Could you check a few things on this model? Use its own coordinates, in mm. Face numbers are marked on the shaded views. A direction names the side the tool comes from. Coordinates: 2 decimals unless noted, no trailing zeros. Loops run counter-clockwise (first coordinate to the right, second up) from the corner with the lowest first, then second, coordinate; pieces in that order, holes last.
1) Imagine slicing it at C-C on y = -9.75. Please give me the cut outline in (x, z), plus the area to 4 significant figures.
2) Imagine slicing it at A-A on y = 0. Please give me the cut outline in (x, z).
3) If I drill on line 1 along Y through (x, z) = (0, 14.5); line 2 along Y through (x, z) = (2.5, 14.5); line 3 along Z through (x, y) = (6.75, -6.5), over which ranges is the centre line in solid material (lowest first)?
4) Imagine slicing it at B-B on z = 4.25. Please give me the cut outline in (x, y).
5) For the marked faces 1 and 2, which set-ups out of +Z, -Z, +X, -X, +Y, -Y let a thin tool reach every point of the face, with its end or its side?
6) Will these pins go through, and if not, where does the flat tip stop? P1, Ø1, axis at x = 4, z = 17, coming from the -Y side; P2, Ø3, axis at x = 6.5, z = 6.5, coming from the +Y side; P3, Ø1, axis at x = -4.5, z = 3, coming from the -Y side; P4, Ø6, axis at x = -0.5, y = -0.5, coming from the +Z side.
7) Imagine slicing it at D-D on x = 7.5. Please give me the cut outline in (y, z).
8) Thinking about a two-plate mould opening in X: for the marked faces 3, 4 and 5, which applies, released by +X, released by -X, zero draft, split by the parting line, or undercut?
```python
from build123d import *

# Parameters (mm, degrees)
BOSS_EXTRUDE1_DEPTH = 7.62
SKETCH2_R           = 6.35
BOSS_EXTRUDE2_DEPTH = 12.7
SKETCH3_R           = 3.81
CUT_EXTRUDE1_DEPTH  = 21.32
CHAMFER1_SIZE       = 1.27


with BuildPart() as part:
    # Sketch1 → Boss-Extrude1 (new body)
    with BuildSketch(Plane.XY):
        Polygon((10.31875, 5.95753309), (0, 11.91506618), (-10.31875, 5.95753309), (-10.31875, -5.95753309), (0, -11.91506618), (10.31875, -5.95753309), align=None)
    extrude(amount=BOSS_EXTRUDE1_DEPTH)

    # Sketch2 → Boss-Extrude2 (add)
    with BuildSketch(Plane.XY.offset(7.62)):
        Circle(SKETCH2_R)
    extrude(amount=BOSS_EXTRUDE2_DEPTH)

    # Sketch3 → Cut-Extrude1 (cut, through all)
    with BuildSketch(Plane.XY.offset(20.32)):
        Circle(SKETCH3_R)
    extrude(amount=-CUT_EXTRUDE1_DEPTH, mode=Mode.SUBTRACT)

    # Chamfer1
    chamfer1_edges = [part.edges().sort_by_distance(p)[0] for p in [
        (-3.81, 0, 0),
        (-3.81, 0, 20.32),
    ]]
    chamfer(chamfer1_edges, length=CHAMFER1_SIZE)


solid = part.part
```
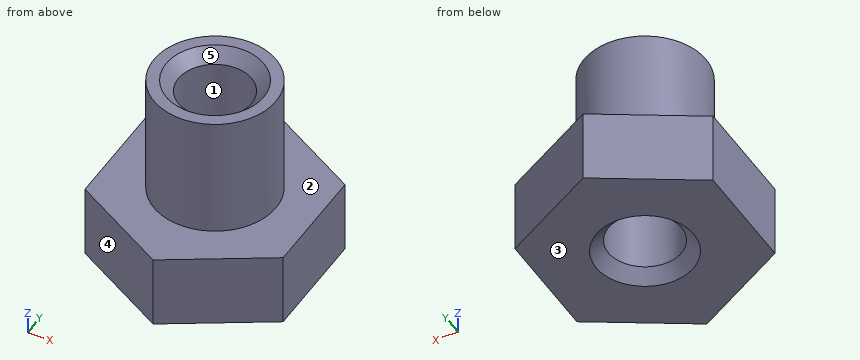
Filled in:
1. outline: (-3.75, 0) - (3.75, 0) - (3.75, 7.62) - (-3.75, 7.62) - close
1. area: 57.15 mm2
2. outline: (-10.32, 0) - (-5.08, 0) - (-3.81, 1.27) - (-3.81, 19.05) - (-5.08, 20.32) - (-6.35, 20.32) - (-6.35, 7.62) - (-10.32, 7.62) - close; (3.81, 1.27) - (5.08, 0) - (10.32, 0) - (10.32, 7.62) - (6.35, 7.62) - (6.35, 20.32) - (5.08, 20.32) - (3.81, 19.05) - close
3. line 1: y = -6.35 to -3.81, 3.81 to 6.35
3. line 2: y = -5.84 to -2.88, 2.88 to 5.84
3. line 3: z = 0 to 7.62
4. outline: (-10.32, -5.96) - (0, -11.92) - (10.32, -5.96) - (10.32, 5.96) - (0, 11.92) - (-10.32, 5.96) - close; hole circle Ø7.62 at (0, 0)
5. face 1: +Z, -Z
5. face 2: +Z
6. P1: stops at y = -5.3
6. P2: stops at y = 9.03
6. P3: stops at y = -9.61
6. P4: passes through
7. outline: (-7.58, 0) - (7.58, 0) - (7.58, 7.62) - (-7.58, 7.62) - close
8. face 3: zero draft
8. face 4: released by -X
8. face 5: undercut
